Read the model definition and answer for the solid it produces. Units are mm, in the model's axes. A direction names the side the tool comes from. Give positions to 0.01 mm unless a question says otherwise; leave off trailing zeros. Order: outer loops, then holes, each group sorted by start corner. A loop starts at its lowest first (then second) coordinate and runs counter-clockwise, first axis right, second up. Notation, with made-up numbers: (8, -23.75) - (53, -23.75) arc R16 ccw to (53, -14.75) - close; hole circle Ø3 at (-36, -14.75). An arc over 180 degrees is marked (long way). Use a Markdown table: item, result. Add a question column.
1. Which of the six approach directions +Z, -Z, +X, -X, +Y, -Y give full straight-line access (tool end or side, diameter ignored) to faces 1 (the flat face through (10, -155, 79)), 2 (the cylindrical face through (5.33, -152.52, 12.46)), 3 (the flat face through (123, -86, 158))?
2. Flat-ended cylindrical pins translate along their axes: P1, Ø4, axis at x = 105, y = -80, coming from the +Z side; P2, Ø1.5, axis at x = 154, y = -154.5, coming from the -Z side; P3, Ø11, axis at x = 66, y = -4, coming from the -Z side. Find the tip coordinate at first contact, or state that the pin passes through.
3. Consider L1, parallel to Y at x = 155, z = 12.65; L2, parallel to X at y = -155, z = 12.35; L3, parallel to Y at x = 105, z = 156. Determine where each line is inside the solid, lowest interval first.
4. A cutting plane is placed at D-D on y = -80. Determine the outline of the cut face in (x, z), and give its area (3 significant figures).
5. A cutting plane is placed at A-A on x = 105. Determine the outline of the cut face in (y, z).
6. A cutting plane is placed at C-C on z = 86.5. Determine the outline of the cut face in (x, y), and give its area (3 significant figures).
7. A cutting plane is placed at B-B on y = -105.5. Determine the outline of the cut face in (x, z), and give its area (3 significant figures).
8. For a pull along Y with two mould halves and no side action, classify faces 4 (the cylindrical face through (2.615, -4.249, 12.465)), 5 (the flat face through (5, -10, 79)), 6 (the flat face through (3, -157, 10)), 7 (the flat face through (80, 0, 151)) as released by +Y, released by -Y, zero draft, split by the parting line, or undercut.
```python
from build123d import *

# Parameters (mm, degrees)
CROQUIS2_W                   = 160
CROQUIS2_H                   = 160
CROQUIS2_W_2                 = 140
CROQUIS2_H_2                 = 140
SALIENTE_EXTRUIR1_DEPTH      = 10
CROQUIS3_W                   = 152
CROQUIS3_H                   = 152
CROQUIS3_W_2                 = 150
CROQUIS3_H_2                 = 150
CROQUIS3_W_3                 = 148
CROQUIS3_H_3                 = 148
CORTAR_EXTRUIR1_DEPTH        = 3.5
CROQUIS4_W                   = 10
CROQUIS4_H                   = 10
SALIENTE_EXTRUIR2_DEPTH      = 140
SALIENTE_EXTRUIR2_DEPTH_BACK = 10
CROQUIS7_W                   = 160
CROQUIS7_H                   = 160
CROQUIS7_W_2                 = 140
CROQUIS7_H_2                 = 140
SALIENTE_EXTRUIR3_DEPTH      = 10
CROQUIS8_W                   = 63
CROQUIS8_H                   = 12
CROQUIS8_R                   = 2.5
SALIENTE_EXTRUIR4_DEPTH      = 5
CROQUIS9_W                   = 10
CROQUIS9_H                   = 160
CORTAR_EXTRUIR2_DEPTH        = 161
CROQUIS10_R                  = 2.5
CORTAR_EXTRUIR3_DEPTH        = 5


with BuildPart() as part:
    # Croquis2 → Saliente-Extruir1 (new body)
    with BuildSketch(Plane.XY):
        with Locations((80, -80)):
            Rectangle(CROQUIS2_W, CROQUIS2_H)
        with Locations((80, -80)):
            Rectangle(CROQUIS2_W_2, CROQUIS2_H_2, mode=Mode.SUBTRACT)
    extrude(amount=SALIENTE_EXTRUIR1_DEPTH)

    # Croquis3 → Cortar-Extruir1 (cut)
    with BuildSketch(Plane.XY.offset(10)):
        with Locations((80, -80)):
            Rectangle(CROQUIS3_W, CROQUIS3_H)
        with Locations((80, -80)):
            Rectangle(CROQUIS3_W_2, CROQUIS3_H_2, mode=Mode.SUBTRACT)
        with Locations((80, -80)):
            Rectangle(CROQUIS3_W_2, CROQUIS3_H_2)
        with Locations((80, -80)):
            Rectangle(CROQUIS3_W_3, CROQUIS3_H_3, mode=Mode.SUBTRACT)
    extrude(amount=-CORTAR_EXTRUIR1_DEPTH, mode=Mode.SUBTRACT)

    # Croquis4 → Saliente-Extruir2 (add, two sides)
    with BuildSketch(Plane.XY.offset(10)) as saliente_extruir2_sk:
        with Locations((5, -5)):
            Rectangle(CROQUIS4_W, CROQUIS4_H)
        with Locations((155, -5)):
            Rectangle(CROQUIS4_W, CROQUIS4_H)
        with Locations((155, -155)):
            Rectangle(CROQUIS4_W, CROQUIS4_H)
        with Locations((5, -155)):
            Rectangle(CROQUIS4_W, CROQUIS4_H)
    extrude(amount=SALIENTE_EXTRUIR2_DEPTH)
    extrude(saliente_extruir2_sk.sketch, amount=-SALIENTE_EXTRUIR2_DEPTH_BACK)

    # Croquis7 → Saliente-Extruir3 (add)
    with BuildSketch(Plane.XY.offset(150)):
        with Locations((80, -80)):
            Rectangle(CROQUIS7_W, CROQUIS7_H)
        with Locations((80, -80)):
            Rectangle(CROQUIS7_W_2, CROQUIS7_H_2, mode=Mode.SUBTRACT)
    extrude(amount=SALIENTE_EXTRUIR3_DEPTH)

    # Croquis8 → Saliente-Extruir4 (add)
    with BuildSketch(Plane.XY.offset(160)):
        with Locations((31.5, -80)):
            Rectangle(CROQUIS8_W, CROQUIS8_H)
        with Locations((55, -80)):
            Circle(CROQUIS8_R, mode=Mode.SUBTRACT)
        with Locations((128.5, -80)):
            Rectangle(CROQUIS8_W, CROQUIS8_H)
        with Locations((105, -80)):
            Circle(CROQUIS8_R, mode=Mode.SUBTRACT)
    extrude(amount=-SALIENTE_EXTRUIR4_DEPTH)

    # Croquis9 → Cortar-Extruir2 (cut, through all)
    with BuildSketch(Plane.ZY):
        with Locations((5, -80)):
            Rectangle(CROQUIS9_W, CROQUIS9_H)
    extrude(amount=-CORTAR_EXTRUIR2_DEPTH, mode=Mode.SUBTRACT)

    # Croquis10 → Cortar-Extruir3 (cut)
    with BuildSketch(Plane(origin=(0, 0, 10), x_dir=(-1, 0, 0), z_dir=(0, 0, -1))):
        with Locations((-155, -155)):
            Circle(CROQUIS10_R)
        with Locations((-5, -5)):
            Circle(CROQUIS10_R)
        with Locations((-155, -5)):
            Circle(CROQUIS10_R)
        with Locations((-5, -155)):
            Circle(CROQUIS10_R)
    extrude(amount=-CORTAR_EXTRUIR3_DEPTH, mode=Mode.SUBTRACT)


solid = part.part
```
Output values:
| question | item | result |
|---|---|---|
| 1 | face 1 | -Z, +Y, -Y |
| 1 | face 2 | -Z |
| 1 | face 3 | +Z, -Z |
| 2 | P1 | through |
| 2 | P2 | z = 15 |
| 2 | P3 | z = 150 |
| 3 | L1 | -160 to -157.5, -152.5 to -150, -10 to -7.5, -2.5 to 0 |
| 3 | L2 | 0 to 2.5, 7.5 to 10, 150 to 152.5, 157.5 to 160 |
| 3 | L3 | -160 to -150, -86 to -82.5, -77.5 to -74, -10 to 0 |
| 4 | outline | (0, 150) - (10, 150) - (10, 155) - (52.5, 155) - (52.5, 160) - (0, 160) - close; (57.5, 155) - (63, 155) - (63, 160) - (57.5, 160) - close; (97, 155) - (102.5, 155) - (102.5, 160) - (97, 160) - close; (107.5, 155) - (150, 155) - (150, 150) - (160, 150) - (160, 160) - (107.5, 160) - close |
| 4 | area | 680 mm² |
| 5 | outline | (-160, 150) - (-150, 150) - (-150, 160) - (-160, 160) - close; (-86, 155) - (-82.5, 155) - (-82.5, 160) - (-86, 160) - close; (-77.5, 155) - (-74, 155) - (-74, 160) - (-77.5, 160) - close; (-10, 150) - (0, 150) - (0, 160) - (-10, 160) - close |
| 6 | outline | (0, -160) - (10, -160) - (10, -150) - (0, -150) - close; (0, -10) - (10, -10) - (10, 0) - (0, 0) - close; (150, -160) - (160, -160) - (160, -150) - (150, -150) - close; (150, -10) - (160, -10) - (160, 0) - (150, 0) - close |
| 6 | area | 400 mm² |
| 7 | outline | (0, 150) - (10, 150) - (10, 160) - (0, 160) - close; (150, 150) - (160, 150) - (160, 160) - (150, 160) - close |
| 7 | area | 200 mm² |
| 8 | face 4 | undercut |
| 8 | face 5 | undercut |
| 8 | face 6 | zero draft |
| 8 | face 7 | released by +Y |
